Source: CAD feature listing. Evaluate the final solid. Frame: model axes, mm. Round coordinates to 2 decimals unless told otherwise and drop trailing zeros. Order: outer loops, then holes, each group sorted by start corner. A loop starts at its lowest first (then second) coordinate and runs counter-clockwise, first axis right, second up. Notation, with made-up numbers: M 76,16.25 L 116,16.25 A31 ccw 116,45.25 Z; hole C -4.75,72.25 d7. An arc over 180 degrees is marked long. Answer as CSV lines item,"result". Start each with the question number.
Item 1: Line query: line 1 (X direction, y = 87.5, z = 3.8); line 2 (Y direction, x = 100.5, z = 2.35); line 3 (X direction, y = 208, z = 2.7). Output: solid intervals per line, ascending. Write a range as [from, to].
Item 2: Section query C-C on y = 184. Return the cut outline in (x, z).
Item 3: Section query A-A on y = 99.5. Return the cut outline in (x, z).
Item 4: Section query B-B on z = 4.25. State how many separate pieces and enclosed holes the cut face has, plus the area to 3 significant figures.
Item 5: First-contact query: P1, Ø3, axis at x = 39.5, z = 3.5, coming from the -Y side; P2, Ø4.5, axis at x = -100.076, y = 63.5, coming from the -Z side; P3, Ø2.5, axis at x = 277.876, y = 63.5, coming from the -Z side; P4, Ø2.5, axis at y = 204, z = 2.5, coming from the +X side. Flat tips, straight axial feed; report the tip coordinate or a pass-through.
Item 6: Section query D-D on x = -76. Return the cut outline in (y, z), plus the area to 3 significant figures.
from build123d import *

# Parameters (mm, degrees)
BOSS_EXTRUDE1_DEPTH = 5.08
SKETCH2_R           = 2
CUT_EXTRUDE1_DEPTH  = 5.08
SKETCH3_R           = 1.905
CUT_EXTRUDE2_DEPTH  = 5.08
SKETCH4_W           = 102.616
SKETCH4_H           = 127
BOSS_EXTRUDE2_DEPTH = 5.08
SKETCH8_W           = 88.9
SKETCH8_H           = 19.05
CUT_EXTRUDE3_DEPTH  = 50.8
SKETCH9_R           = 1.4224
CUT_EXTRUDE4_DEPTH  = 10.16


with BuildPart() as part:
    # Sketch1 → Boss-Extrude1 (new body)
    with BuildSketch(Plane.XY):
        Polygon((0, 0), (0, 228.6), (177.8, 228.6), (177.8, 0), (142.24, 0), (142.24, 114.3), (35.56, 114.3), (35.56, 0), align=None)
    extrude(amount=BOSS_EXTRUDE1_DEPTH)

    # Sketch2 → Cut-Extrude1 (cut)
    with BuildSketch(Plane(origin=(0, 0, 0), x_dir=(-1, 0, 0), z_dir=(0, 0, -1))):
        with Locations((-21.59, 111.071616712)):
            Circle(SKETCH2_R)
        with Locations((-3.811028038, 111.071616712)):
            Circle(SKETCH2_R)
        with Locations((-21.59, 75.511616712)):
            Circle(SKETCH2_R)
        with Locations((-3.811028038, 75.320420507)):
            Circle(SKETCH2_R)
    extrude(amount=-CUT_EXTRUDE1_DEPTH, mode=Mode.SUBTRACT)

    # Sketch3 → Cut-Extrude2 (cut)
    with BuildSketch(Plane(origin=(0, 0, 0), x_dir=(-1, 0, 0), z_dir=(0, 0, -1))):
        with Locations((-151.12245979, 123.444)):
            Circle(SKETCH3_R)
        with Locations((-151.12245979, 87.884)):
            Circle(SKETCH3_R)
    extrude(amount=-CUT_EXTRUDE2_DEPTH, mode=Mode.SUBTRACT)

    # Sketch4 → Boss-Extrude2 (add)
    with BuildSketch(Plane(origin=(0, 0, 0), x_dir=(-1, 0, 0), z_dir=(0, 0, -1))):
        with Locations((51.308, 63.5)):
            Rectangle(SKETCH4_W, SKETCH4_H)
        with Locations((-229.108, 63.5)):
            Rectangle(SKETCH4_W, SKETCH4_H)
    extrude(amount=-BOSS_EXTRUDE2_DEPTH)

    # Sketch8 → Cut-Extrude3 (cut)
    with BuildSketch(Plane(origin=(0, 0, 0), x_dir=(-1, 0, 0), z_dir=(0, 0, -1))):
        with Locations((-88.9, 203.073)):
            Rectangle(SKETCH8_W, SKETCH8_H)
    extrude(amount=-CUT_EXTRUDE3_DEPTH, mode=Mode.SUBTRACT)

    # Sketch9 → Cut-Extrude4 (cut)
    with BuildSketch(Plane(origin=(0, 0, 0), x_dir=(-1, 0, 0), z_dir=(0, 0, -1))):
        with Locations((100.076, 12.7)):
            Circle(SKETCH9_R)
        with Locations((100.076, 63.5)):
            Circle(SKETCH9_R)
        with Locations((100.076, 114.3)):
            Circle(SKETCH9_R)
        with Locations((-277.876, 63.5)):
            Circle(SKETCH9_R)
        with Locations((-277.876, 114.3)):
            Circle(SKETCH9_R)
        with Locations((-277.876, 12.7)):
            Circle(SKETCH9_R)
    extrude(amount=-CUT_EXTRUDE4_DEPTH, mode=Mode.SUBTRACT)


solid = part.part
Results:
1,line 1,"[-102.62, 35.56], [142.24, 149.26], [152.99, 280.42]"
1,line 2,"[114.3, 193.55], [212.6, 228.6]"
1,line 3,"[0, 44.45], [133.35, 177.8]"
2,outline,"M 0,0 L 177.8,0 L 177.8,5.08 L 0,5.08 Z"
3,outline,"M -102.62,0 L 35.56,0 L 35.56,5.08 L -102.62,5.08 Z; M 142.24,0 L 280.42,0 L 280.42,5.08 L 142.24,5.08 Z"
4,separate pieces,"1"
4,enclosed holes,"13"
4,area,"52,700 mm^2"
5,P1,"y = 114.3"
5,P2,"z = 0"
5,P3,"through"
5,P4,"x = 177.8"
6,outline,"M 0,0 L 127,0 L 127,5.08 L 0,5.08 Z"
6,area,"645 mm^2"
